Autodesk Inventor part; units mm, degrees
ref_plane "YZ Plane" through (0, 0, 0) normal (1, 0, 0) x (0, 1, 0)
ref_plane "XZ Plane" through (0, 0, 0) normal (0, 1, 0) x (-1, 0, 0)
ref_plane "XY Plane" through (0, 0, 0) normal (0, 0, 1) x (1, 0, 0)
sketch "Sketch1" plane through (0, 0, 0) normal (0, 0, 1) x (1, 0, 0)
  line L0 (-10.8185, 29.4098) -> (2.1815, 29.4098)
  line L1 (2.1815, 29.4098) -> (2.1815, -6.8902)
  line L2 (2.1815, -6.8902) -> (-10.8185, -6.8902)
  line L3 (-10.8185, -6.8902) -> (-10.8185, 29.4098)
  point P0 (0, 0)
  dimension "d0" = 13
  dimension "d1" = 36.3
extrude "Extrusion1" add sketch "Sketch1" along normal blind 6
sketch "Sketch2" plane through (0, 0, 6) normal (0, 0, 1) x (1, 0, 0)
  line L0 (2.1815, 29.4098) -> (-10.8185, 29.4098)
  line L1 (-10.8185, 29.4098) -> (-10.8185, -6.8902)
  line L2 (-10.8185, -6.8902) -> (2.1815, -6.8902)
  line L3 (2.1815, -6.8902) -> (2.1815, 29.4098)
  line L4 (2.1815, -0.7902) -> (-10.8185, -0.7902)
  line L5 (-10.8185, 29.4098) -> (-10.8185, -6.8902)
  line L6 (-10.8185, 5.2098) -> (2.1815, 5.2098)
  line L7 (2.1815, -6.8902) -> (2.1815, 29.4098)
  line L8 (-10.8185, 17.3098) -> (2.1815, 17.3098)
  line L9 (-10.8185, 23.3098) -> (2.1815, 23.3098)
  point P0 (0, 0)
  dimension "d4" = 6.1
  dimension "d5" = 6.1
  dimension "d6" = 12.1
  dimension "d7" = 12.1
  dimension "d8" = 36.3
extrude "Extrusion2" add sketch "Sketch2" along normal blind 17.1 contours L3 L9 L1 L0 | L3 L6 L1 L8 | L3 L2 L1 L4
chamfer "Chamfer1" distance 0.3 angle 45 16 edges at (-10.8185, 29.4098, 11.55) (-10.8185, 23.3098, 14.55) (-10.8185, 17.3098, 14.55) (2.1815, 17.3098, 14.55) (2.1815, 5.2098, 14.55) (-10.8185, 5.2098, 14.55) (-10.8185, -0.7902, 14.55) (2.1815, -0.7902, 14.55) (-10.8185, -6.8902, 11.55) (2.1815, -6.8902, 11.55) (2.1815, 29.4098, 11.55) (2.1815, 23.3098, 14.55) (-10.8185, 11.2598, 0) (2.1815, 11.2598, 0) (-4.3185, 29.4098, 0) (-4.3185, -6.8902, 0)
equation "\"d5\" = d4"
equation "\"d7\" = -0.5 * d6 + 0.5 * d8"
properties part number "COTS_GENERIC_Transformer_Core" material "Stainless Steel"
The model under review builds one solid part; all positions refer to its coordinate system, in mm. A direction names the side the tool comes from. Round coordinates to 2 decimals unless told otherwise and drop trailing zeros. Write each loop counter-clockwise with the first axis right and the second up, starting at its lowest first coordinate (ties: lowest second). Pieces come first, ordered by that corner, then holes.
(1) We need section C-C on y = 20. Give the boundary of the cut face in (x, z).
(2) Wall thickness on L1, parallel to Y at x = -6, z = 20.5; L2, parallel to Z at x = 0, y = 3: over which ranges is each line inside the solid? List them lowest first.
(3) Insertion check: pin 1 (3.5 mm diameter, centred on x = -7, y = 3, fed in from +Z). The pin has a flat end and moves straight along its axis. Give the tip position at first contact, or say it passes through.
(4) Mouldability with a two-part tool opening along Y and no side actions: class faces 3 (the flat face through (-4, 23.31, 14)), 4 (the flat face through (-4, 11, 23.1)), 5 (the flat face through (-4, 29.41, 12)) as +Y half, -Y half, draft (parallel to the pull), parting line (faces both ways), or undercut.
(5) Machinability: for faces 1 (the flat face through (-4, 17.31, 14)), 2 (the flat face through (-4, -6.89, 12)), which of the approach directions +Z, -Z, +X, -X, +Y, -Y give a long, thin tool a straight path to every point of the face, cutting with its end or side? Answer none if there is none.
(6) We need section B-B on x = -3.5. Give the boundary of the cut face in (y, z), and give its area (3 significant figures).
(7) We need section A-A on z = 18. Give the boundary of the cut face in (x, y), and give its area (3 significant figures).
Findings below:
1. outline: (-10.82, 0.3) - (-10.52, 0) - (1.88, 0) - (2.18, 0.3) - (2.18, 6) - (-10.82, 6) - close
2. L1: y = -6.89 to -0.79, 5.21 to 17.31, 23.31 to 29.41
2. L2: z = 0 to 6
3. pin 1: stops at z = 6
4. face 3: undercut
4. face 4: draft
4. face 5: +Y half
5. face 1: +Z, +X, -X
5. face 2: +Z, -Z, +X, -X, -Y
6. outline: (-6.89, 0.3) - (-6.59, 0) - (29.11, 0) - (29.41, 0.3) - (29.41, 23.1) - (23.31, 23.1) - (23.31, 6) - (17.31, 6) - (17.31, 23.1) - (5.21, 23.1) - (5.21, 6) - (-0.79, 6) - (-0.79, 23.1) - (-6.89, 23.1) - close
6. area: 633 mm2
7. outline: (-10.82, -6.59) - (-10.52, -6.89) - (1.88, -6.89) - (2.18, -6.59) - (2.18, -1.09) - (1.88, -0.79) - (-10.52, -0.79) - (-10.82, -1.09) - close; (-10.82, 5.51) - (-10.52, 5.21) - (1.88, 5.21) - (2.18, 5.51) - (2.18, 17.01) - (1.88, 17.31) - (-10.52, 17.31) - (-10.82, 17.01) - close; (-10.82, 23.61) - (-10.52, 23.31) - (1.88, 23.31) - (2.18, 23.61) - (2.18, 29.11) - (1.88, 29.41) - (-10.52, 29.41) - (-10.82, 29.11) - close
7. area: 315 mm2
